```python
from build123d import *

# Parameters (mm, degrees)
F0_R     = 6.35
F0_R_2   = 4.7625
F1_DEPTH = 63.5
F2_DEPTH = 50.8
F4_DEPTH = 25.4


with BuildPart() as f1:
    # F0 (on Top) → F1 (new body)
    with BuildSketch(Plane.XY):
        Circle(F0_R)
        Circle(F0_R_2, mode=Mode.SUBTRACT)
        Circle(F0_R_2)
    extrude(amount=-F1_DEPTH)

    # F0 (on Top) → F2 (cut)
    with BuildSketch(Plane.XY):
        Circle(F0_R_2)
    extrude(amount=-F2_DEPTH, mode=Mode.SUBTRACT)

    # F3 (on Right) → F4 (cut)
    with BuildSketch(Plane.YZ):
        with BuildLine():
            Line((2.54, -30.48), (2.54, -5.08))
            ThreePointArc((2.54, -5.08), (0, -2.54), (-2.54, -5.08))
            Line((-2.54, -5.08), (-2.54, -30.48))
            ThreePointArc((-2.54, -30.48), (0, -33.02), (2.54, -30.48))
        make_face()
    extrude(amount=-F4_DEPTH, mode=Mode.SUBTRACT)


solid = f1.part
```
Can you work these out from the model? Positions are in its coordinate system, mm. A direction names the side the tool comes from. Round coordinates to 2 decimals unless told otherwise and drop trailing zeros. Loops run counter-clockwise (first coordinate to the right, second up) from the corner with the lowest first, then second, coordinate; pieces in that order, holes last.
Item 1: Suppose I cut it at C-C, the plane y = -3.5. Write out the boundary of the cut face in (x, z).
Item 2: Suppose I cut it at B-B, the plane x = 0. Write out the boundary of the cut face in (y, z), then the cut area to 3 significant figures.
Item 3: If we mould it in two halves opening along Z, with no side actions, what happens to faces 4 (the flat face through (0, 0, -63.5)), 5 (the flat face through (-5, 2.54, -18)), 6 (the flat face through (1, 5, 0))? For each: +Z half, -Z half, draft (parallel to the pull), parting line (faces both ways), or undercut.
Item 4: Suppose I cut it at A-A, the plane y = 0. Write out the boundary of the cut face in (x, z).
Item 5: Will these pins go through, and if not, where does the flat tip stop? pin 1 Ø1.4 at (x, z) = (-5, -14) entering from -Y; pin 2 Ø0.9 at (x, z) = (-5.5, -12.5) entering from +Y.
Item 6: Please list where these lines run through material, in increasing order: L1, parallel to Y at x = 0, z = -32.5; L2, parallel to X at y = 0, z = -20.5; L3, parallel to Y at x = 3, z = -8.5.
Item 7: Which directions (+Z, -Z, +X, -X, +Y, -Y) give clear straight access to the entire face, cutting with the end or side of a thin tool? Please do faces 1 (the cylindrical face through (4.543, 1.431, -25.044)), 2 (the cylindrical face through (6.057, 1.907, -31.306)), 3 (the cylindrical face through (-5.17, 0.06, -2.54)).
Reported:
1. outline: (-5.3, -63.5) - (5.3, -63.5) - (5.3, 0) - (3.23, 0) - (3.23, -50.8) - (-3.23, -50.8) - (-3.23, 0) - (-5.3, 0) - close
2. outline: (-6.35, -63.5) - (6.35, -63.5) - (6.35, 0) - (4.76, 0) - (4.76, -50.8) - (-4.76, -50.8) - (-4.76, 0) - (-6.35, 0) - close
2. area: 323 mm2
3. face 4: -Z half
3. face 5: undercut
3. face 6: +Z half
4. outline: (-6.35, -63.5) - (6.35, -63.5) - (6.35, 0) - (4.76, 0) - (4.76, -50.8) - (-4.76, -50.8) - (-4.76, -33.02) - (-6.35, -33.02) - close; (-6.35, -2.54) - (-4.76, -2.54) - (-4.76, 0) - (-6.35, 0) - close
5. pin 1: stops at y = -4.67
5. pin 2: stops at y = 3.85
6. L1: y = -6.35 to -4.76, 4.76 to 6.35
6. L2: x = 4.76 to 6.35
6. L3: y = -5.6 to -3.7, 3.7 to 5.6
7. face 1: +Z
7. face 2: +Z, -Z
7. face 3: -X
